The listing builds one solid part. Answer for the finished solid, in the listing's coordinates (mm). A direction names the side the tool comes from. Give positions to 0.01 mm unless a question says otherwise; leave off trailing zeros. Order: outer loops, then holes, each group sorted by start corner. A loop starts at its lowest first (then second) coordinate and runs counter-clockwise, first axis right, second up.
```python
from build123d import *

# Parameters (mm, degrees)
SKETCH1_W           = 30
SKETCH1_H           = 10
SKETCH1_R           = 1.7
BOSS_EXTRUDE1_DEPTH = 4
BOSS_EXTRUDE2_START = -13.4
BOSS_EXTRUDE2_DEPTH = 13.4
SKETCH3_R           = 1.25
CUT_EXTRUDE1_DEPTH  = 2
FILLET1_R           = 1
CHAMFER1_SIZE       = 0.6


with BuildPart() as part:
    # Sketch1 → Boss-Extrude1 (new body)
    with BuildSketch(Plane.XY):
        with Locations((34.05, 0)):
            Rectangle(SKETCH1_W, SKETCH1_H)
        with Locations((44.05, 0)):
            Circle(SKETCH1_R, mode=Mode.SUBTRACT)
        with Locations((24.05, 0)):
            Circle(SKETCH1_R, mode=Mode.SUBTRACT)
    extrude(amount=BOSS_EXTRUDE1_DEPTH)

    # Sketch2 → Boss-Extrude2 (add)
    with BuildSketch(Plane.ZY.offset(-27.35).offset(BOSS_EXTRUDE2_START)):
        Polygon((21.756367983, -8.555), (4, -8.555), (4, -5), (0, -5), (0, -12.555), (21.756367983, -12.555), align=None)
    extrude(amount=BOSS_EXTRUDE2_DEPTH)

    # Sketch3 → Cut-Extrude1 (cut)
    with BuildSketch(Plane(origin=(0, -8.555, 0), x_dir=(1, 0, 0), z_dir=(0, 1, 0))):
        with Locations((30.17, -18.316367983)):
            Circle(SKETCH3_R)
        with Locations((37.93, -18.316367983)):
            Circle(SKETCH3_R)
    extrude(amount=-CUT_EXTRUDE1_DEPTH, mode=Mode.SUBTRACT)

    # Fillet1
    fillet1_edges = [part.edges().sort_by_distance(p)[0] for p in [
        (19.05, 0, 4),
        (23.2, -5, 4),
        (44.9, -5, 4),
        (34.05, -8.555, 21.756367983),
        (34.05, -12.555, 21.756367983),
        (27.35, -10.555, 21.756367983),
        (27.35, -8.555, 12.878183991),
        (27.35, -6.7775, 4),
        (27.35, -5, 2),
        (27.35, -12.555, 10.878183991),
        (40.75, -10.555, 21.756367983),
        (40.75, -12.555, 10.878183991),
        (40.75, -5, 2),
        (40.75, -6.7775, 4),
        (40.75, -8.555, 12.878183991),
        (49.05, 0, 4),
        (49.05, -5, 2),
        (19.05, -5, 2),
        (19.05, 5, 2),
        (49.05, 5, 2),
        (34.05, 5, 4),
    ]]
    fillet(fillet1_edges, radius=FILLET1_R)

    # Chamfer1
    chamfer1_edges = [part.edges().sort_by_distance(p)[0] for p in [
        (42.35, 0, 0),
        (22.35, 0, 0),
        (23.2, -5, 0),
        (40.75, -8.7775, 0),
        (19.05, 0, 0),
        (27.35, -8.7775, 0),
        (34.05, 5, 0),
        (49.05, 0, 0),
        (44.9, -5, 0),
        (34.05, -12.555, 0),
        (19.342893219, -4.707106781, 0),
        (19.342893219, 4.707106781, 0),
        (48.757106781, 4.707106781, 0),
        (48.757106781, -4.707106781, 0),
        (40.457106781, -12.262106781, 0),
        (27.642893219, -12.262106781, 0),
        (41.042893219, -5.292893219, 0),
        (27.057106781, -5.292893219, 0),
    ]]
    chamfer(chamfer1_edges, length=CHAMFER1_SIZE)


solid = part.part
```
1) Find section C-C (x = 35). Write down the section's boundary in (y, z) (3 decimals), then the cut area to 3 significant figures.
Geometry says:
outline: (-12.555, 0.6) - (-11.955, 0) - (4.4, 0) - (5, 0.6) - (5, 3) arc R1 ccw to (4, 4) - (-8.555, 4) - (-8.555, 20.756) arc R1 ccw to (-9.555, 21.756) - (-11.555, 21.756) arc R1 ccw to (-12.555, 20.756) - close
area: 140 mm2
2) Find section A-A (x = 44.05). Write down the section's boundary in (y, z).
Geometry says:
outline: (-5, 0.6) - (-4.4, 0) - (-2.3, 0) - (-1.7, 0.6) - (-1.7, 4) - (-4, 4) arc R1 ccw to (-5, 3) - close; (1.7, 0.6) - (2.3, 0) - (4.4, 0) - (5, 0.6) - (5, 3) arc R1 ccw to (4, 4) - (1.7, 4) - close
3) Straight lines are drawn through the part: probe 1 along Z at (x, y) = (30.17, -9.8); probe 2 along X at (y, z) = (1.5, 3.75); probe 3 along Z at (x, y) = (37.5, 4). For each, find the intervals that lie inside material, in ascending order.
Geometry says:
probe 1: z = 0 to 17.07, 19.57 to 21.76
probe 2: x = 19.39 to 23.25, 24.85 to 43.25, 44.85 to 48.71
probe 3: z = 0 to 4
4) Given P1, Ø5, axis at y = -9, z = 19.5, coming from the +X side; P2, Ø1.5, axis at y = -6.5, z = 5.5, coming from the +X side; P3, Ø8, axis at y = -6.5, z = 19, coming from the -X side; P4, Ø3.5, axis at x = 31.5, z = 12.5, coming from the +Y side (3 decimals), each flat-ended and moving along its own axis, determine where each tip first touches the part or whether it passes through.
Geometry says:
P1: stops at x = 40.75
P2: passes through
P3: stops at x = 27.35
P4: stops at y = -8.555
5) Find section B-B (y = 0). Write down the section's boundary in (x, z), then the cut area to 3 significant figures.
Geometry says:
outline: (19.05, 0.6) - (19.65, 0) - (21.75, 0) - (22.35, 0.6) - (22.35, 4) - (20.05, 4) arc R1 ccw to (19.05, 3) - close; (25.75, 0.6) - (26.35, 0) - (41.75, 0) - (42.35, 0.6) - (42.35, 4) - (25.75, 4) - close; (45.75, 0.6) - (46.35, 0) - (48.45, 0) - (49.05, 0.6) - (49.05, 3) arc R1 ccw to (48.05, 4) - (45.75, 4) - close
area: 91.3 mm2
6) A tool of negligible diameter and unlimited length cuts with its end or side. For faces 1 (the cylindrical face through (38.6, -9.54, 17.26)), 2 (the flat face through (23, -5, 2)), 3 (the flat face through (34, -8.555, 12)), 4 (the cylindrical face through (23.244, -4.715, 3.699)), from which of +Z, -Z, +X, -X, +Y, -Y can it reach the whole face along a straight path? Write none if from no direction.
Geometry says:
face 1: +Y
face 2: +Z, -Z, -X, -Y
face 3: +Z, +X, -X, +Y
face 4: +Z, -X, -Y
7) Find section D-D (z = 16.25). Write down the section's boundary in (x, y) (3 decimals), then the cut area to 3 significant figures.
Geometry says:
outline: (27.35, -11.555) arc R1 ccw to (28.35, -12.555) - (39.75, -12.555) arc R1 ccw to (40.75, -11.555) - (40.75, -9.555) arc R1 ccw to (39.75, -8.555) - (28.35, -8.555) arc R1 ccw to (27.35, -9.555) - close
area: 52.7 mm2
8) For a pull along Y with two mould halves and no side action, classify faces 5 (the cylindrical face through (22.35, 0.07, 2.28)), 6 (the cylindrical face through (33.97, -8.84, 21.456)), 7 (the flat face through (34, -11, 21.756)), 8 (the cylindrical face through (45.67, 0.51, 2.28)) as +Y half, -Y half, draft (parallel to the pull), parting line (faces both ways), or undercut.
Geometry says:
face 5: undercut
face 6: +Y half
face 7: draft
face 8: undercut
